Read the model definition and answer for the solid it produces. Units are mm, in the model's axes. Face numbers are marked on the shaded views. A direction names the side the tool comes from. Give positions to 0.01 mm unless a question says otherwise; leave off trailing zeros. Loops run counter-clockwise (first coordinate to the right, second up) from the corner with the lowest first, then second, coordinate; pieces in that order, holes last. Notation, with made-up numbers: M 83,49.25 L 134,49.25 A8 ccw 134,64.25 Z; hole C 46,-10 d7. An arc over 180 degrees is marked long. Return JSON: item names as keys, results as strings. Group by question number.
Autodesk Inventor part; units mm, degrees
ref_plane "YZ Plane" through (0, 0, 0) normal (1, 0, 0) x (0, 1, 0)
ref_plane "XZ Plane" through (0, 0, 0) normal (0, 1, 0) x (-1, 0, 0)
ref_plane "XY Plane" through (0, 0, 0) normal (0, 0, 1) x (1, 0, 0)
sketch "Sketch1" plane through (0, 0, 0) normal (0, 0, 1) x (1, 0, 0)
  line L0 (-31, 6.1) -> (0, 6.1)
  line L1 (0, 6.1) -> (31, 6.1)
  line L2 (0, 10.5424) -> (0, 0) construction
  line L3 (31, 9.75) -> (31, 6.1)
  line L4 (77, 9.75) -> (77, 0)
  line L5 (46.4247, 9.75) -> (46.4247, 4.1503)
  line L6 (46.4247, 4.1503) -> (48.4247, 4.1503)
  line L7 (48.4247, 4.1503) -> (48.4247, 9.75)
  line L8 (31, 9.75) -> (46.4247, 9.75) construction
  line L9 (31, 9.75) -> (46.4247, 9.75)
  line L10 (62.7124, 9.75) -> (62.7124, 9.1289)
  line L11 (62.7124, 9.1289) -> (62.9117, 9.1289)
  line L12 (62.9117, 9.1289) -> (62.9117, 9.75)
  line L13 (48.4247, 9.75) -> (62.7124, 9.75) construction
  line L14 (62.9117, 9.75) -> (77, 9.75) construction
  line L15 (48.4247, 9.75) -> (62.7124, 9.75)
  line L16 (62.9117, 9.75) -> (77, 9.75)
  line L17 (-31, 8.1) -> (-60.2, 8.1)
  line L18 (-60.2, 8.1) -> (-60.2, 0)
  line L19 (-31, 8.1) -> (-31, 6.1)
  line L20 (-60.2, 4.875) -> (-63.45, 4.875)
  line L21 (-66.7, 0) -> (-60.2, 0)
  line L22 (-63.45, 4.875) -> (-63.45, 2.7274)
  line L23 (-63.45, 2.7274) -> (-65.075, 2.7274)
  line L24 (-65.075, 2.7274) -> (-65.075, 1.425)
  line L25 (-65.075, 1.425) -> (-66.7, 1.425)
  line L26 (-66.7, 1.425) -> (-66.7, 0)
  line L27 (-60.2, 0) -> (77, 0)
  line L28 (-95.44, 0) -> (105.74, 0)
  dimension "d1" = 31
  dimension "d2" = 31
  dimension "d3" = 6.1
  dimension "d4" = 46
  dimension "d6" = 2
  dimension "d7" = 29.2
  dimension "d8" = 8.1
  dimension "d10" = 1.425
  dimension "d11" = 6.5
revolve "Revolution1" add sketch "Sketch1" angle 360 about axis through (-10, 0, 0) along (1, 0, 0)
properties part number "PH Monitor"
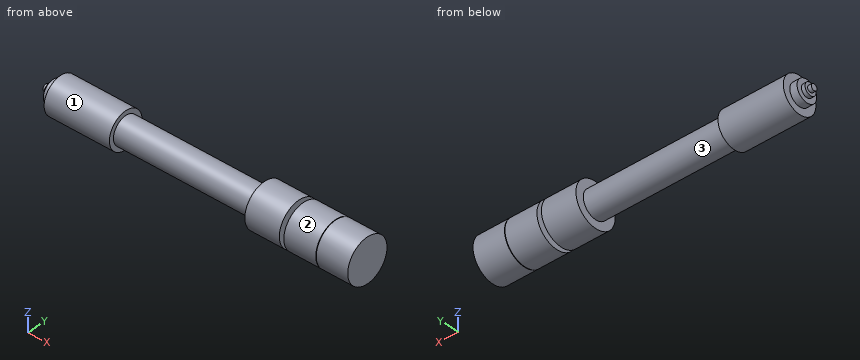
1. Find section A-A (x = -47). Write down the section's boundary in (y, z).
2. Straight lines are drawn through the part: line 1 along X through (y, z) = (-2.25, -6.75); line 2 along X through (y, z) = (3.25, 4.75); line 3 along X through (y, z) = (5.75, -6.5). For each, find the intervals that lie inside material, in ascending order.
3. For the marked faces 1, 2 and 3, determine the directions among +Z, -Z, +X, -X, +Y, -Y from which every point of the face is accessible in a straight line to the end or side of a thin tool.
4. Find section B-B (x = -8). Write down the section's boundary in (y, z).
5. Flat-ended cylindrical pins translate along their axes: P1, Ø1, axis at x = 10, z = -3, coming from the +Y side; P2, Ø4, axis at y = 1, z = 6.5, coming from the -X side; P3, Ø1.5, axis at x = 44, z = 6, coming from the +Y side. Find the tip coordinate at first contact, or state that the pin passes through.
Result:
{
 "1": {"outline": "C 0,0 d16.2"},
 "2": {"line 1": "x = -60.2 to -31, 31 to 46.42, 48.42 to 77", "line 2": "x = -60.2 to 46.42, 48.42 to 77", "line 3": "x = 31 to 46.42, 48.42 to 77"},
 "3": {"face 1": "-X", "face 2": "+X, -X", "face 3": "none"},
 "4": {"outline": "C 0,0 d12.2"},
 "5": {"P1": "stops at y = 5.56", "P2": "stops at x = -63.45", "P3": "stops at y = 8.22"}
}
